from build123d import *

# Parameters (mm, degrees)
SKETCH_1_R      = 1.55
SKETCH_1_R_2    = 1.3
EXTRUDE_1_DEPTH = 2


with BuildPart() as part:
    # 草图1 → 凸台-拉伸1 (new body)
    with BuildSketch(Plane(origin=(0, 0, 0), x_dir=(1, 0, 0), z_dir=(0, 1, 0))):
        with BuildLine():
            Line((-30.40246304, 52.857720294), (-32.037278544, 51.028700347))
            ThreePointArc((-32.037278544, 51.028700347), (-34.725061467, 48.527352956), (-37.824815498, 46.559501145))
            ThreePointArc((-37.824815498, 46.559501145), (-39.603619628, 44.736066121), (-39.92091739, 42.208541335))
            ThreePointArc((-39.92091739, 42.208541335), (-36.468177596, 39.027493268), (-32.370509151, 41.318692124))
            ThreePointArc((-32.370509151, 41.318692124), (-31.135199663, 43.325028618), (-29.464750167, 44.986646546))
            Line((-29.464750167, 44.986646546), (-12.33593628, 58.408952508))
            ThreePointArc((-12.33593628, 58.408952508), (0, 62.666504283), (12.33593628, 58.408952508))
            Line((12.33593628, 58.408952508), (29.464750167, 44.986646546))
            ThreePointArc((29.464750167, 44.986646546), (31.135199663, 43.325028618), (32.370509151, 41.318692124))
            ThreePointArc((32.370509151, 41.318692124), (36.468177596, 39.027493268), (39.92091739, 42.208541335))
            ThreePointArc((39.92091739, 42.208541335), (39.603619628, 44.736066121), (37.824815498, 46.559501145))
            ThreePointArc((37.824815498, 46.559501145), (34.725061467, 48.527352956), (32.037278544, 51.028700347))
            Line((32.037278544, 51.028700347), (30.40246304, 52.857720294))
            ThreePointArc((30.40246304, 52.857720294), (23.129287971, 62.333031959), (17.34800881, 72.785659285))
            Line((17.34800881, 72.785659285), (15.34970392, 77.137234504))
            ThreePointArc((15.34970392, 77.137234504), (14.242702771, 78.410741128), (12.62341972, 78.885286238))
            Line((12.62341972, 78.885286238), (-12.62341972, 78.885286238))
            ThreePointArc((-12.62341972, 78.885286238), (-14.242702771, 78.410741128), (-15.34970392, 77.137234504))
            Line((-15.34970392, 77.137234504), (-17.34800881, 72.785659285))
            ThreePointArc((-17.34800881, 72.785659285), (-23.129287971, 62.333031959), (-30.40246304, 52.857720294))
        make_face()
        with Locations(Location((-36, 43, 0), (0, 0, 270))):
            Circle(SKETCH_1_R, mode=Mode.SUBTRACT)
        with Locations(Location((36, 43, 0), (0, 0, 270))):
            Circle(SKETCH_1_R, mode=Mode.SUBTRACT)
        with Locations(Location((-12.15, 64.075512735, 0), (0, 0, 270))):
            Circle(SKETCH_1_R_2, mode=Mode.SUBTRACT)
        with Locations(Location((-12.15, 76.105512735, 0), (0, 0, 270))):
            Circle(SKETCH_1_R_2, mode=Mode.SUBTRACT)
        with Locations(Location((12.15, 64.075512735, 0), (0, 0, 270))):
            Circle(SKETCH_1_R_2, mode=Mode.SUBTRACT)
        with Locations(Location((12.15, 76.105512735, 0), (0, 0, 270))):
            Circle(SKETCH_1_R_2, mode=Mode.SUBTRACT)
    extrude(amount=EXTRUDE_1_DEPTH)


solid = part.part
Part model, mm, in its own coordinate system. A direction names the side the tool comes from. Coordinates: 2 decimals unless noted, no trailing zeros. Loops run counter-clockwise (first coordinate to the right, second up) from the corner with the lowest first, then second, coordinate; pieces in that order, holes last. Notation, with made-up numbers: M 64.25,-25 L 97.25,-25 A22 ccw 97.25,12 Z; hole C 38.25,69 d8. An arc over 180 degrees is marked long. Use a Markdown table: item, result. Add a question column.
Q1. Pin check, flat tips, straight feed: P1, Ø4, axis at x = 12.15, z = -64.08, coming from the +Y side; P2, Ø1, axis at y = 2, z = -51, coming from the +X side; P3, Ø1, axis at y = 1.5, z = -64, coming from the +X side; P4, Ø1, axis at x = 14, y = 1.5, coming from the +Z side. Stop position of each tip, or through.
Q2. Which spindle directions (+Z, -Z, +X, -X, +Y, -Y) get a long thin tool onto all of the face, cutting with end or side? Do faces 1 (the flat face through (0, 2, -65)), 2 (the flat face through (20.78, 0.99, -51.79)). Say none if no direction does.
Q3. Cut at A-A (y = 1.7). Write the cut outline in (x, z).
Q4. Cut at C-C (x = 36). Write the cut outline in (y, z).
Q5. Probe L1, parallel to X at y = 1, z = -63.5; L2, parallel to X at y = 1.3, z = -63; L3, parallel to X at y = 0.75, z = -56. List the from-to ranges inside material, lowest first.
Q6. Mould opens along X. For faces 3 (the flat face through (0, 1, -78.885)), 4 (the cylindrical face through (14.26, 0.99, -78.4)), 5 (the flat face through (-16.335, 0.986, -74.992)), 6 (the cylindrical face through (11.652, 0.986, -74.905)) say: +X half, -X half, draft (parallel to the pull), parting line (faces both ways), or undercut.
Q7. Cut at B-B (z = -49.5). Write the cut outline in (x, y).
Q8. Cut at D-D (z = -43). Write the cut outline in (x, y).
Worked out:
| question | item | result |
|---|---|---|
| 1 | P1 | stops at y = 2 |
| 1 | P2 | stops at x = 32.53 |
| 1 | P3 | stops at x = 22.38 |
| 1 | P4 | stops at z = -56.71 |
| 2 | face 1 | +Z, -Z, +X, -X, +Y |
| 2 | face 2 | +Z, +Y, -Y |
| 3 | outline | M -37.82,-46.56 A20 cw -32.04,-51.03 L -30.4,-52.86 A80 cw -17.35,-72.79 L -15.35,-77.14 A3 ccw -12.62,-78.89 L 12.62,-78.89 A3 ccw 15.35,-77.14 L 17.35,-72.79 A80 cw 30.4,-52.86 L 32.04,-51.03 A20 cw 37.82,-46.56 A4 ccw long 32.37,-41.32 A10 cw 29.46,-44.99 L 12.34,-58.41 A20 cw -12.34,-58.41 L -29.46,-44.99 A10 cw -32.37,-41.32 A4 ccw long Z; hole C -36,-43 d3.1; hole C -12.15,-76.11 d2.6; hole C -12.15,-64.08 d2.6; hole C 12.15,-76.11 d2.6; hole C 12.15,-64.08 d2.6; hole C 36,-43 d3.1 |
| 4 | outline | M 0,-47.62 L 2,-47.62 L 2,-44.55 L 0,-44.55 Z; M 0,-41.45 L 2,-41.45 L 2,-39 L 0,-39 Z |
| 5 | L1 | x = -22.38 to -13.32, -10.98 to 10.98, 13.32 to 22.38 |
| 5 | L2 | x = -22.7 to -12.88, -11.42 to 11.42, 12.88 to 22.7 |
| 5 | L3 | x = -27.74 to -15.41, 15.41 to 27.74 |
| 6 | face 3 | draft |
| 6 | face 4 | +X half |
| 6 | face 5 | -X half |
| 6 | face 6 | undercut |
| 7 | outline | M -33.56,0 L -23.71,0 L -23.71,2 L -33.56,2 Z; M 23.71,0 L 33.56,0 L 33.56,2 L 23.71,2 Z |
| 8 | outline | M -40,0 L -37.55,0 L -37.55,2 L -40,2 Z; M -34.45,0 L -31.38,0 L -31.38,2 L -34.45,2 Z; M 31.38,0 L 34.45,0 L 34.45,2 L 31.38,2 Z; M 37.55,0 L 40,0 L 40,2 L 37.55,2 Z |
